Design review of the part built by this model. Coordinates are the model's own, in mm. Face numbers are marked on the shaded views. A direction names the side the tool comes from. Coordinates: 2 decimals unless noted, no trailing zeros. Loops run counter-clockwise (first coordinate to the right, second up) from the corner with the lowest first, then second, coordinate; pieces in that order, holes last. Notation, with made-up numbers: (4.25, 68.5) -> (45.25, 68.5) arc R28 cw to (45.25, 95.5) -> close; hole circle Ø8 at (-0.5, 42.25). An arc over 180 degrees is marked (long way). Answer as a JSON object with one key per item and string values.
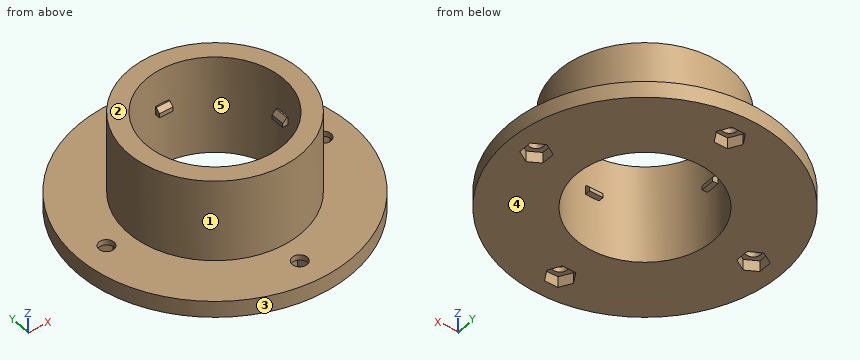
```python
from build123d import *

# Parameters (mm, degrees)
SZKIC1_R                    = 50
DODANIE_WYCI_GNI_CIE1_DEPTH = 6
SZKIC2_R                    = 31.5
DODANIE_WYCI_GNI_CIE2_DEPTH = 30
SZKIC3_R                    = 25
WYTNIJ_WYCI_GNI_CIE1_DEPTH  = 80.3473377
SZKIC4_W                    = 5
SZKIC4_H                    = 5
DODANIE_WYCI_GNI_CIE3_DEPTH = 3
SFAZOWANIE2_START           = -1
SFAZOWANIE2_OUTLINE_W       = 5
SFAZOWANIE2_OUTLINE_H       = 2.121320343
SFAZOWANIE2_DEPTH           = 2.060660172
SZYK_KO_OWY3_COUNT          = 4
WYTNIJ_WYCI_GNI_CIE2_DEPTH  = 4
SZKIC6_R                    = 2.75
WYTNIJ_WYCI_GNI_CIE3_DEPTH  = 78.614431648


with BuildPart() as part:
    # Szkic1 → Dodanie-wyci_gni_cie1 (new body)
    with BuildSketch(Plane.XY):
        Circle(SZKIC1_R)
    extrude(amount=DODANIE_WYCI_GNI_CIE1_DEPTH)

    # Szkic2 → Dodanie-wyci_gni_cie2 (add)
    with BuildSketch(Plane.XY.offset(6)):
        Circle(SZKIC2_R)
    extrude(amount=DODANIE_WYCI_GNI_CIE2_DEPTH)

    # Szkic3 → Wytnij-wyci_gni_cie1 (cut, through all)
    with BuildSketch(Plane.XY.offset(36)):
        Circle(SZKIC3_R)
    extrude(amount=-WYTNIJ_WYCI_GNI_CIE1_DEPTH, mode=Mode.SUBTRACT)

    # Szkic4 → Dodanie-wyci_gni_cie3 (add)
    with BuildSketch(Plane.XY.offset(20)):
        with Locations((0, 25.5)):
            Rectangle(SZKIC4_W, SZKIC4_H)
    dodanie_wyci_gni_cie3 = extrude(amount=DODANIE_WYCI_GNI_CIE3_DEPTH)

    # Sfazowanie2: read off the stored shape, not the designer's step
    # Sfazowanie2 outline → Sfazowanie2 (cut)
    with BuildSketch(Plane(origin=(0, 0, 0), x_dir=(1, 0, 0), z_dir=(0, 0.707106781186548, -0.707106781186547)).offset(SFAZOWANIE2_START)):
        with Locations((0, -32.526911935)):
            Rectangle(SFAZOWANIE2_OUTLINE_W, SFAZOWANIE2_OUTLINE_H)
    sfazowanie2 = extrude(amount=SFAZOWANIE2_DEPTH, mode=Mode.SUBTRACT)

    # Szyk ko_owy3: Dodanie-wyci_gni_cie3, Sfazowanie2 ×4 about axis
    szyk_ko_owy3_axis = Axis((0, 0, 0), (0, 0, 1))
    add([dodanie_wyci_gni_cie3.rotate(szyk_ko_owy3_axis, i * 360 / SZYK_KO_OWY3_COUNT) for i in range(1, SZYK_KO_OWY3_COUNT)])
    add([sfazowanie2.rotate(szyk_ko_owy3_axis, i * 360 / SZYK_KO_OWY3_COUNT) for i in range(1, SZYK_KO_OWY3_COUNT)], mode=Mode.SUBTRACT)

    # Szkic5 → Wytnij-wyci_gni_cie2 (cut)
    with BuildSketch(Plane(origin=(0, 0, 0), x_dir=(-1, 0, 0), z_dir=(0, 0, -1))):
        Polygon((40, -4.907477288), (44.25, -2.453738644), (44.25, 2.453738644), (40, 4.907477288), (35.75, 2.453738644), (35.75, -2.453738644), align=None)
        Polygon((4.907477288, 40), (2.453738644, 44.25), (-2.453738644, 44.25), (-4.907477288, 40), (-2.453738644, 35.75), (2.453738644, 35.75), align=None)
        Polygon((-4.907477288, -40), (-2.453738644, -44.25), (2.453738644, -44.25), (4.907477288, -40), (2.453738644, -35.75), (-2.453738644, -35.75), align=None)
        Polygon((-40, 4.907477288), (-44.25, 2.453738644), (-44.25, -2.453738644), (-40, -4.907477288), (-35.75, -2.453738644), (-35.75, 2.453738644), align=None)
    extrude(amount=-WYTNIJ_WYCI_GNI_CIE2_DEPTH, mode=Mode.SUBTRACT)

    # Szkic6 → Wytnij-wyci_gni_cie3 (cut, through all)
    with BuildSketch(Plane(origin=(0, 0, 4), x_dir=(-1, 0, 0), z_dir=(0, 0, -1))):
        with Locations((0, 40)):
            Circle(SZKIC6_R)
        with Locations((40, 0)):
            Circle(SZKIC6_R)
        with Locations((0, -40)):
            Circle(SZKIC6_R)
        with Locations((-40, 0)):
            Circle(SZKIC6_R)
    extrude(amount=-WYTNIJ_WYCI_GNI_CIE3_DEPTH, mode=Mode.SUBTRACT)


solid = part.part
```
1) Add section A-A, the plane y = -15.5. Give the boundary of the cut face in (x, z), and give its area (3 significant figures).
Completed:
{"outline": "(-47.54, 0) -> (-19.62, 0) -> (-19.62, 36) -> (-27.42, 36) -> (-27.42, 6) -> (-47.54, 6) -> close; (19.62, 0) -> (47.54, 0) -> (47.54, 6) -> (27.42, 6) -> (27.42, 36) -> (19.62, 36) -> close", "area": "804 mm²"}
2) Add section C-C, the plane z = 9. Give the boundary of the cut face in (x, y).
Completed:
{"outline": "circle Ø63 at (0, 0); hole circle Ø50 at (0, 0)"}
3) For the marked faces 1 and 2, list the 3-axis set-ups (+Z, -Z, +X, -X, +Y, -Y) from which the entire face can be reached by the end or side of a thin tool; tool diameter is ignored.
Completed:
{"face 1": "+Z", "face 2": "+Z, +X, -X, +Y, -Y"}
4) Wall thickness on probe 1 along Y at (x, z) = (0, 5); probe 2 along X at (y, z) = (-1, 15.5); probe 3 along Z at (x, y) = (-20.5, 34): over which ranges is each line inside the solid? List them lowest first.
Completed:
{"probe 1": "-50 to -42.75, -37.25 to -25, 25 to 37.25, 42.75 to 50", "probe 2": "-31.48 to -24.98, 24.98 to 31.48", "probe 3": "0 to 6"}
5) Add section D-D, the plane x = 0. Count the separate pieces of the cut face and the enclosed holes in it, and give its area (3 significant figures).
Completed:
{"separate pieces": "4", "enclosed holes": "0", "area": "610 mm²"}
6) Clearance check with flat-ended pins moving along their axes: pin 1 Ø5 at (x, y) = (-16.5, -37.5) entering from +Z; pin 2 Ø7 at (x, y) = (-0.5, 40) entering from -Z; pin 3 Ø0.5 at (x, z) = (-1, 20.5) entering from +Y. State where each tip first meets the part, or that it passes through.
Completed:
{"pin 1": "z = 6", "pin 2": "z = 4", "pin 3": "y = 31.49"}
7) The part is to be moulded in two halves that separate along X. For the marked faces 3, 4 and 5, say which applies: pulls with the +X half, pulls with the -X half, needs draft (parallel to the pull), parting line crosses it, or undercut.
Completed:
{"face 3": "parting line crosses it", "face 4": "needs draft", "face 5": "undercut"}
